```python
from build123d import *

# Parameters (mm, degrees)
EXTRUDE_1_DEPTH     = 3
SKETCH_2_R          = 1.35
CUT_EXTRUDE_1_DEPTH = 2.444444444
SKETCH_3_R          = 1.6
SKETCH_3_R_2        = 1.35
CUT_EXTRUDE_3_DEPTH = 96.756657889


with BuildPart() as part:
    # 草图1 → 凸台-拉伸1 (new body)
    with BuildSketch(Plane.XY.offset(3)):
        with BuildLine():
            Line((-60.832535173, 7.514094179), (-91.218664305, 7.514094179))
            ThreePointArc((-91.218664305, 7.514094179), (-95.218664305, 3.514094179), (-91.218664305, -0.485905821))
            Line((-91.218664305, -0.485905821), (-60.531573746, -0.485905821))
            ThreePointArc((-60.531573746, -0.485905821), (-56.589491156, -2.306217172), (-52.451603626, -0.990377005))
            Line((-52.451603626, -0.990377005), (-50.420982545, -0.990377005))
            Line((-50.420982545, -0.990377005), (23.816560918, 0.467808699))
            Line((23.816560918, 0.467808699), (23.856567982, 0.468594524))
            ThreePointArc((23.856567982, 0.468594524), (27.777723532, 4.507000717), (23.778016459, 8.467622986))
            Line((23.778016459, 8.467622986), (-52.596358319, 8.467622986))
            ThreePointArc((-52.596358319, 8.467622986), (-56.905640848, 9.642312032), (-60.832535173, 7.514094179))
        make_face()
    extrude(amount=-EXTRUDE_1_DEPTH)

    # 草图2 → 切除-拉伸1 (cut)
    with BuildSketch(Plane.XY.offset(3)):
        with Locations(Location((23.77801746, 4.467622995, 0), (0, 0, 180))):
            Circle(SKETCH_2_R)
    extrude(amount=-CUT_EXTRUDE_1_DEPTH, mode=Mode.SUBTRACT)

    # 草图3 → 切除-拉伸3 (cut, through all)
    with BuildSketch(Plane(origin=(0, 0, 0), x_dir=(-1, 0, 0), z_dir=(0, 0, -1))):
        with Locations(Location((-23.778017455, 4.467823177, 0), (0, 0, 180))):
            Circle(SKETCH_3_R)
        with Locations((56.215610459, 3.6821226)):
            Circle(SKETCH_3_R)
        with Locations((91.218664305, 3.514094179)):
            Circle(SKETCH_3_R_2)
    extrude(amount=-CUT_EXTRUDE_3_DEPTH, mode=Mode.SUBTRACT)


solid = part.part
```
Could you check a few things on this model? Use its own coordinates, in mm. A direction names the side the tool comes from. Coordinates: 2 decimals unless noted, no trailing zeros. Write each loop counter-clockwise with the first axis right and the second up, starting at its lowest first coordinate (ties: lowest second). Pieces come first, ordered by that corner, then holes. Notation, with made-up numbers: (-20, 82.25) - (7, 82.25) arc R36 cw to (7, 118.25) - close; hole circle Ø6 at (23, 9.25). An arc over 180 degrees is marked (long way). Use a Markdown table: item, result.
Q1. Imagine slicing it at A-A (z = 2.3). List the corners of the cut face in (x, y) for me, and give its area (3 significant figures).
Geometry check:
| item | result |
|---|---|
| outline | (-91.22, -0.49) - (-60.53, -0.49) arc R6 ccw to (-52.45, -0.99) - (-50.42, -0.99) - (23.86, 0.47) arc R4 ccw to (23.78, 8.47) - (-52.6, 8.47) arc R6 ccw to (-60.83, 7.51) - (-91.22, 7.51) arc R4 ccw to start; hole circle Ø2.7 at (-91.22, 3.51); hole circle Ø3.2 at (-56.22, 3.68); hole circle Ø3.2 at (23.78, 4.47) |
| area | 1,030 mm2 |
Q2. I'm going to push flat-ended pins straight in: pin 1 Ø1.5 at (x, z) = (-80.5, 2) entering from +Y; pin 2 Ø5 at (x, y) = (-63.5, -1) entering from -Z; pin 3 Ø2 at (x, y) = (-91.22, 3.51) entering from -Z; pin 4 Ø1.5 at (x, z) = (-73, 1.5) entering from -Y. Where does each tip first touch, or does it pass through?
Geometry check:
| item | result |
|---|---|
| pin 1 | stops at y = 7.51 |
| pin 2 | stops at z = 0 |
| pin 3 | passes through |
| pin 4 | stops at y = -0.49 |
Q3. Imagine slicing it at B-B (x = -71). List the corners of the cut face in (y, z) for me, and give its area (3 significant figures).
Geometry check:
| item | result |
|---|---|
| outline | (-0.49, 0) - (7.51, 0) - (7.51, 3) - (-0.49, 3) - close |
| area | 24.0 mm2 |
Q4. Which directions (+Z, -Z, +X, -X, +Y, -Y) give clear straight access to the entire face, cutting with the end or side of a thin tool? Please do faces 1 (the flat face through (-14, 8.468, 2)), 2 (the flat face through (-51, -0.99, 2)), 3 (the flat face through (-76, -0.486, 2)).
Geometry check:
| item | result |
|---|---|
| face 1 | +Z, -Z, +X, +Y |
| face 2 | +Z, -Z, +X, -Y |
| face 3 | +Z, -Z, -X, -Y |
Q5. Imagine slicing it at C-C (x = 20). List the corners of the cut face in (y, z) for me, and give its area (3 significant figures).
Geometry check:
| item | result |
|---|---|
| outline | (0.39, 0) - (8.47, 0) - (8.47, 3) - (0.39, 3) - close |
| area | 24.2 mm2 |
Q6. Please list where these lines run through material, in increasing order: L1, parallel to X at y = 4.75, z = 2.2; L2, parallel to X at y = 3, z = 0.4; L3, parallel to X at y = 2.5, z = 2.55.
Geometry check:
| item | result |
|---|---|
| L1 | x = -95.02 to -91.76, -90.68 to -57.41, -55.02 to 22.2, 25.35 to 27.77 |
| L2 | x = -95.19 to -92.47, -89.97 to -57.66, -54.77 to 23.14, 24.41 to 27.5 |
| L3 | x = -95.09 to -92.11, -90.33 to -57.29, -55.14 to 27.26 |
Q7. Thinking about a two-plate mould opening in Y: for faces 4 (the flat face through (-76, 7.514, 2)), 5 (the flat face through (-35, 4, 3)), 6 (the cylindrical face through (-89.87, 3.57, 1.48)), which applies, +Y half, -Y half, draft (parallel to the pull), parting line (faces both ways), or undercut?
Geometry check:
| item | result |
|---|---|
| face 4 | +Y half |
| face 5 | draft |
| face 6 | undercut |
